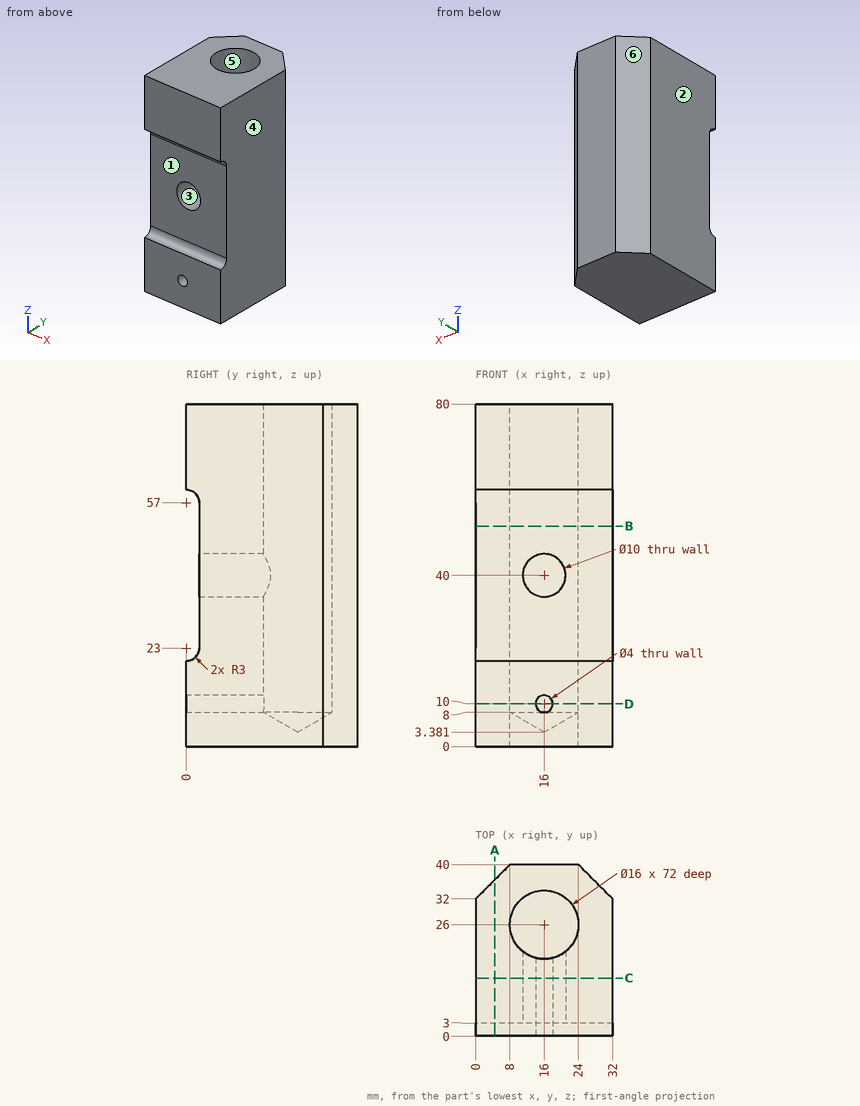
Answer from the drawing. Dimensions are ordinates in mm from the lowest x, y and z of the part. A direction names the side the tool comes from. Round coordinates to 2 decimals unless told otherwise and drop trailing zeros. Loops run counter-clockwise (first coordinate to the right, second up) from the corner with the lowest first, then second, coordinate; pieces in that order, holes last.
(1) The part is cut by section D-D, the plane z = 10. Give the vertices of the cut face in (x, y), and give its area (3 significant figures).
Computed values:
outline: (0, 0) - (14, 0) - (14, 18.25) arc R8 cw (long way) to (18, 18.25) - (18, 0) - (32, 0) - (32, 32) - (24, 40) - (8, 40) - (0, 32) - close
area: 943 mm2
(2) Each of these flat-tipped pins is pushed along its axis until it touches: P1, Ø12, axis at x = 17, y = 13, coming from the -Z side; P2, Ø3.5, axis at x = 16, z = 10, coming from the -Y side; P3, Ø9.5, axis at x = 16, y = 26, coming from the +Z side; P4, Ø4, axis at x = 21.5, z = 41, coming from the -Y side. Where does it stop, or does it pass through?
Computed values:
P1: stops at z = 0
P2: stops at y = 33.81
P3: stops at z = 6.12
P4: stops at y = 3
(3) For the marked faces 1, 2 and 3, determine the directions among +Z, -Z, +X, -X, +Y, -Y from which every point of the face is accessible in a straight line to the end or side of a thin tool.
Computed values:
face 1: +X, -X, -Y
face 2: +Z, -Z, -X, +Y, -Y
face 3: -Y
(4) The part is cut by section A-A, the plane x = 4.5. Give the vertices of the cut face in (y, z), and give its area (3 significant figures).
Computed values:
outline: (0, 0) - (36.5, 0) - (36.5, 80) - (0, 80) - (0, 60) arc R3 cw to (3, 57) - (3, 23) arc R3 cw to (0, 20) - close
area: 2,800 mm2
(5) Find the intervals of material crossed by L1, parallel to Z at x = 16, y = 15.5; L2, parallel to X at y = 7, z = 10; L3, parallel to Y at x = 20.5, z = 7.5 (1 decimal), in increasing order.
Computed values:
L1: z = 0 to 8, 12 to 35, 45 to 80
L2: x = 0 to 14, 18 to 32
L3: y = 0 to 20.5, 31.5 to 40
(6) The mould has two halves that part along Y. Classify the marked faces 4, 5 and 6: pulls with the +Y half, pulls with the -Y half, needs draft (parallel to the pull), parting line crosses it, or undercut.
Computed values:
face 4: needs draft
face 5: undercut
face 6: pulls with the +Y half
(7) The part is cut by section C-C, the plane y = 13.5. Give the vertices of the cut face in (x, z).
Computed values:
outline: (0, 0) - (32, 0) - (32, 80) - (0, 80) - close; hole circle Ø10 at (16, 40); hole circle Ø4 at (16, 10)
(8) The part is cut by section B-B, the plane z = 51.5. Give the vertices of the cut face in (x, y).
Computed values:
outline: (0, 3) - (32, 3) - (32, 32) - (24, 40) - (8, 40) - (0, 32) - close; hole circle Ø16 at (16, 26)
